```python
from build123d import *

# Parameters (mm, degrees)
SKETCH2_W               = 250
SKETCH2_H               = 150
BOSS_EXTRUDE1_DEPTH     = 3
SKETCH3_W               = 10
SKETCH3_H               = 3.3
CUT_EXTRUDE1_DEPTH      = 146.804663849
LPATTERN1_COUNT         = 2
LPATTERN1_PITCH         = 20.5
SKETCH4_W               = 10
SKETCH4_H               = 10
CUT_EXTRUDE2_DEPTH      = 146.804663849
MIRROR1_COPY_1_SKETCH_W = 10
MIRROR1_COPY_1_SKETCH_H = 3.3
MIRROR1_COPY_1_DEPTH    = 146.804663849
MIRROR2_COPY_1_SKETCH_W = 10
MIRROR2_COPY_1_SKETCH_H = 3.3
MIRROR2_COPY_1_DEPTH    = 146.804663849
MIRROR2_COPY_2_SKETCH_W = 10
MIRROR2_COPY_2_SKETCH_H = 3.3
MIRROR2_COPY_2_DEPTH    = 146.804663849
MIRROR2_COPY_3_SKETCH_W = 10
MIRROR2_COPY_3_SKETCH_H = 10
MIRROR2_COPY_3_DEPTH    = 146.804663849
MIRROR2_COPY_4_SKETCH_W = 10
MIRROR2_COPY_4_SKETCH_H = 3.3
MIRROR2_COPY_4_DEPTH    = 146.804663849
SKETCH6_R               = 1.5
CUT_EXTRUDE4_DEPTH      = 146.804663849


with BuildPart() as part:
    # Sketch2 → Boss-Extrude1 (new body)
    with BuildSketch(Plane.XY):
        Rectangle(SKETCH2_W, SKETCH2_H)
    extrude(amount=BOSS_EXTRUDE1_DEPTH)

    # Sketch3 → Cut-Extrude1 (cut, symmetric)
    with BuildSketch(Plane(origin=(0, 0, 0), x_dir=(-1, 0, 0), z_dir=(0, 0, -1))):
        with Locations((-90, 73.35)):
            Rectangle(SKETCH3_W, SKETCH3_H)
    cut_extrude1 = extrude(amount=CUT_EXTRUDE1_DEPTH, both=True, mode=Mode.SUBTRACT)

    # LPattern1: Cut-Extrude1 ×2
    with Locations(*[(0, -i * LPATTERN1_PITCH, 0) for i in range(1, LPATTERN1_COUNT)]):
        add(cut_extrude1, mode=Mode.SUBTRACT)

    # Sketch4 → Cut-Extrude2 (cut, through all)
    with BuildSketch(Plane(origin=(0, 0, 0), x_dir=(-1, 0, 0), z_dir=(0, 0, -1))):
        with Locations((-73, 60)):
            Rectangle(SKETCH4_W, SKETCH4_H)
    cut_extrude2 = extrude(amount=-CUT_EXTRUDE2_DEPTH, mode=Mode.SUBTRACT)

    # Mirror1: Cut-Extrude1, Cut-Extrude2 across plane
    add(cut_extrude1.mirror(Plane.ZX), mode=Mode.SUBTRACT)
    add(cut_extrude2.mirror(Plane.ZX), mode=Mode.SUBTRACT)

    # Mirror1 copy 1 sketch → Mirror1 copy 1 (cut, symmetric)
    with BuildSketch(Plane(origin=(0, 20.5, 0), x_dir=(-1, 0, 0), z_dir=(0, 0, -1))):
        with Locations((-90, -73.35)):
            Rectangle(MIRROR1_COPY_1_SKETCH_W, MIRROR1_COPY_1_SKETCH_H)
    extrude(amount=MIRROR1_COPY_1_DEPTH, both=True, mode=Mode.SUBTRACT)

    # Mirror2: Cut-Extrude1, Cut-Extrude2 across plane
    add(cut_extrude1.mirror(Plane(origin=(0, 0, 0), x_dir=(0, 0, 1), z_dir=(1, 0, 0))), mode=Mode.SUBTRACT)
    add(cut_extrude2.mirror(Plane(origin=(0, 0, 0), x_dir=(0, 0, 1), z_dir=(1, 0, 0))), mode=Mode.SUBTRACT)

    # Mirror2 copy 1 sketch → Mirror2 copy 1 (cut, symmetric)
    with BuildSketch(Plane(origin=(0, -20.5, 0), x_dir=(1, 0, 0), z_dir=(0, 0, -1))):
        with Locations((-90, -73.35)):
            Rectangle(MIRROR2_COPY_1_SKETCH_W, MIRROR2_COPY_1_SKETCH_H)
    extrude(amount=MIRROR2_COPY_1_DEPTH, both=True, mode=Mode.SUBTRACT)

    # Mirror2 copy 2 sketch → Mirror2 copy 2 (cut, symmetric)
    with BuildSketch(Plane(origin=(0, 0, 0), x_dir=(1, 0, 0), z_dir=(0, 0, -1))):
        with Locations((-90, 73.35)):
            Rectangle(MIRROR2_COPY_2_SKETCH_W, MIRROR2_COPY_2_SKETCH_H)
    extrude(amount=MIRROR2_COPY_2_DEPTH, both=True, mode=Mode.SUBTRACT)

    # Mirror2 copy 3 sketch → Mirror2 copy 3 (cut, through all)
    with BuildSketch(Plane(origin=(0, 0, 0), x_dir=(1, 0, 0), z_dir=(0, 0, -1))):
        with Locations((-73, 60)):
            Rectangle(MIRROR2_COPY_3_SKETCH_W, MIRROR2_COPY_3_SKETCH_H)
    extrude(amount=-MIRROR2_COPY_3_DEPTH, mode=Mode.SUBTRACT)

    # Mirror2 copy 4 sketch → Mirror2 copy 4 (cut, symmetric)
    with BuildSketch(Plane(origin=(0, 20.5, 0), x_dir=(1, 0, 0), z_dir=(0, 0, -1))):
        with Locations((-90, 73.35)):
            Rectangle(MIRROR2_COPY_4_SKETCH_W, MIRROR2_COPY_4_SKETCH_H)
    extrude(amount=MIRROR2_COPY_4_DEPTH, both=True, mode=Mode.SUBTRACT)

    # Sketch6 → Cut-Extrude4 (cut, symmetric)
    with BuildSketch(Plane(origin=(0, 0, 0), x_dir=(-1, 0, 0), z_dir=(0, 0, -1))):
        with Locations((-117.5, 15)):
            Circle(SKETCH6_R)
    cut_extrude4 = extrude(amount=CUT_EXTRUDE4_DEPTH, both=True, mode=Mode.SUBTRACT)

    # Mirror3: Cut-Extrude4 across plane
    add(cut_extrude4.mirror(Plane.ZX), mode=Mode.SUBTRACT)


solid = part.part
```
Work out the finished part from the listing and answer in its coordinate system (mm). Coordinates: 2 decimals unless noted, no trailing zeros. Answer as a JSON object with one key per item and string values.
Q1. Given pin 1 Ø1.5 at (x, z) = (-89, 0.5) entering from -Y; pin 2 Ø2.5 at (x, y) = (117.5, 15) entering from -Z, each flat-ended and moving along its own axis, determine where each tip first touches the part or whether it passes through.
Results list:
{"pin 1": "stops at y = -71.7", "pin 2": "passes through"}
Q2. Consider L1, parallel to Y at x = 117.5, z = 1.1; L2, parallel to Y at x = 87, z = 1.5; L3, parallel to X at y = -52, z = 0.4. Determine where each line is inside the solid, lowest interval first. Write a range as from..to.
Results list:
{"L1": "y = -75..-16.5, -13.5..13.5, 16.5..75", "L2": "y = -71.7..-54.5, -51.2..51.2, 54.5..71.7", "L3": "x = -125..-95, -85..85, 95..125"}
Q3. Find section A-A (z = 2). State how many separate pieces and enclosed holes the cut face has, plus the area to 3 significant figures.
Results list:
{"separate pieces": "1", "enclosed holes": "10", "area": "36,800 mm^2"}
